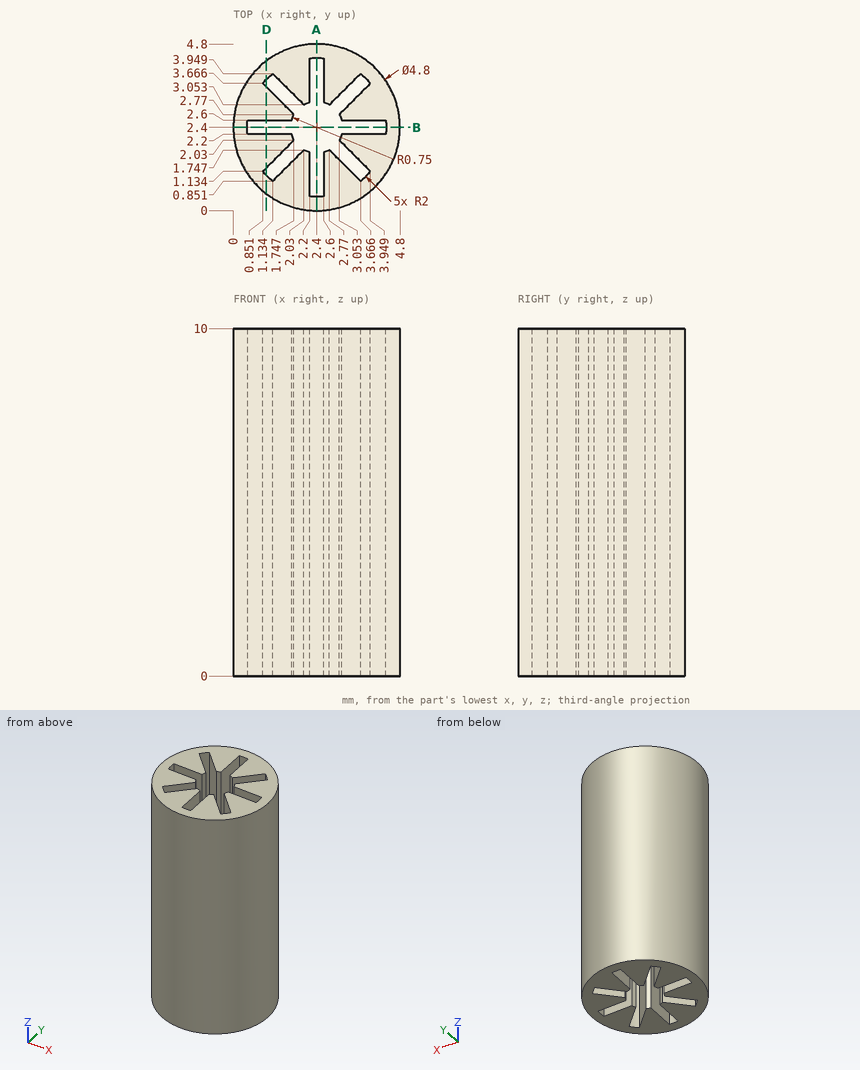
Print and shaded views of the part. All mm, measured from the part's lowest x, y and z. Round coordinates to 2 decimals unless told otherwise and drop trailing zeros. Write each loop counter-clockwise with the first axis right and the second up, starting at its lowest first coordinate (ties: lowest second). Pieces come first, ordered by that corner, then holes. Notation, with made-up numbers: (13.25, -1.75) - (35.25, -1.75) arc R24 cw to (35.25, 30.25) - close; hole circle Ø3 at (62, -19). An arc over 180 degrees is marked (long way). One line per question, with ' | ' between items.
1. Band-saw the part on D-D, the plane x = 0.95. Write the cut outline in (y, z).
Results are:
outline: (0.49, 0) - (1.02, 0) - (1.02, 10) - (0.49, 10) - close; (1.23, 0) - (2.2, 0) - (2.2, 10) - (1.23, 10) - close; (2.6, 0) - (3.57, 0) - (3.57, 10) - (2.6, 10) - close; (3.78, 0) - (4.31, 0) - (4.31, 10) - (3.78, 10) - close
2. Drop flat-ended pins along their axis: pin 1 Ø0.6 at (y, z) = (4, 6) entering from +X; pin 2 Ø1 at (x, z) = (1.5, 8) entering from -Y; pin 3 Ø1.4 at (y, z) = (1, 5.5) entering from -X (1 decimal). Give the stop position or say it passes through.
Results are:
pin 1: x = 4.42 | pin 2: y = 0.03 | pin 3: x = 0.1
3. Drill centre lines: line 1 along X through (y, z) = (3.55, 1.5) (1 decimal); line 2 along X through (y, z) = (3.4, 9.25) (1 decimal); line 3 along Y through (x, z) = (2.5, 6.5). Where is each one in solid material? Low to high. Write a range as from..to.
Results are:
line 1: 0.3..1, 1.5..2.2, 2.6..3.3, 3.8..4.5 | line 2: 0.2..1.1, 1.7..2.2, 2.6..3.1, 3.7..4.6 | line 3: 0..0.4, 4.4..4.8
4. Band-saw the part on A-A, the plane x = 2.4. Write the cut outline in (y, z).
Results are:
outline: (0, 0) - (0.4, 0) - (0.4, 10) - (0, 10) - close; (4.4, 0) - (4.8, 0) - (4.8, 10) - (4.4, 10) - close
